Work out the finished part from the listing and answer in its coordinate system (mm). A direction names the side the tool comes from. Coordinates: 2 decimals unless noted, no trailing zeros. Order: outer loops, then holes, each group sorted by start corner. A loop starts at its lowest first (then second) coordinate and runs counter-clockwise, first axis right, second up. Notation, with made-up numbers: (5.5, -1) -> (11.5, -1) arc R13 cw to (11.5, 14) -> close; hole circle Ø4 at (58, 78.5). An arc over 180 degrees is marked (long way). Answer as CSV lines item,"result". Start each with the question number.
Item 1: For a pull along X with two mould halves and no side action, classify faces 3 (the face through (-46.315, 35, 3)), 4 (the face through (-43.315, 35, 4)), 5 (the face through (-42.315, 35, 4)), 6 (the face through (-43, 36, 6)) as pulls with the +X half, pulls with the -X half, needs draft (parallel to the pull), parting line crosses it, or undercut.
Item 2: Straight lines are drawn through the part: L1, parallel to X at y = 36, z = 5.55; L2, parallel to Z at x = -41.5, y = 36. For each, find the intervals that lie inside material, in ascending order.
Item 3: Section A-A (z = 5.5) is taken. Write down the section's boundary in (x, y), then the cut area to 3 significant figures.
Item 4: Which of the six approach directions +Z, -Z, +X, -X, +Y, -Y give full straight-line access (tool end or side, diameter ignored) to faces 1 (the face through (-35.815, 35, 4)), 2 (the face through (-32.815, 35, 3))?
Item 5: This flat-tipped pin is pushed along its axis until it touches: pin 1 Ø0.9 at (x, y) = (-41.5, 30) entering from +Z. Where does it stop, or does it pass through?
Item 6: Section B-B (y = 48.5) is taken. Write down the section's boundary in (x, z), then the cut area to 4 significant figures.
Item 7: Section C-C (x = -42) is taken. Write down the section's boundary in (y, z), then the cut area to 3 significant figures.
```python
from build123d import *

# Parameters (mm, degrees)
F0_W     = 100
F0_H     = 100
F1_DEPTH = 6
F2_W     = 2
F2_H     = 100
F2_W_2   = 1.75
F2_W_3   = 1.5
F2_W_4   = 1.25
F2_W_5   = 1
F3_DEPTH = 3.5
F4_W     = 86.5
F4_H     = 100
F5_DEPTH = 25
F6_W     = 13.5
F6_H     = 70
F7_DEPTH = 25


with BuildPart() as f1:
    # F0 (on Top) → F1 (new body)
    with BuildSketch(Plane.XY):
        with Locations((3.685346, 0.65935)):
            Rectangle(F0_W, F0_H)
    extrude(amount=F1_DEPTH)

    # F2 (on face) → F3 (cut)
    with BuildSketch(Plane.XY.offset(6)):
        with Locations((-44.314654, 0.65935)):
            Rectangle(F2_W, F2_H)
        with Locations((-41.439654, 0.65935)):
            Rectangle(F2_W_2, F2_H)
        with Locations((-38.814654, 0.65935)):
            Rectangle(F2_W_3, F2_H)
        with Locations((-36.439654, 0.65935)):
            Rectangle(F2_W_4, F2_H)
        with Locations((-34.314654, 0.65935)):
            Rectangle(F2_W_5, F2_H)
    extrude(amount=-F3_DEPTH, mode=Mode.SUBTRACT)

    # F4 (on face) → F5 (cut)
    with BuildSketch(Plane.XY.offset(6)):
        with Locations((10.435346, 0.65935)):
            Rectangle(F4_W, F4_H)
    extrude(amount=-F5_DEPTH, mode=Mode.SUBTRACT)

    # F6 (on face) → F7 (cut)
    with BuildSketch(Plane(origin=(0, 0, 0), x_dir=(1, 0, 0), z_dir=(0, 0, -1))):
        with Locations((-39.564654, 14.34065)):
            Rectangle(F6_W, F6_H)
    extrude(amount=-F7_DEPTH, mode=Mode.SUBTRACT)


solid = f1.part
```
Checked values:
1,face 3,"pulls with the -X half"
1,face 4,"undercut"
1,face 5,"undercut"
1,face 6,"needs draft"
2,L1,"x = -46.31 to -45.31, -43.31 to -42.31, -40.56 to -39.56, -38.06 to -37.06, -35.81 to -34.81, -33.81 to -32.81"
2,L2,"z = 0 to 2.5"
3,outline,"(-46.31, 20.66) -> (-45.31, 20.66) -> (-45.31, 50.66) -> (-46.31, 50.66) -> close; (-43.31, 20.66) -> (-42.31, 20.66) -> (-42.31, 50.66) -> (-43.31, 50.66) -> close; (-40.56, 20.66) -> (-39.56, 20.66) -> (-39.56, 50.66) -> (-40.56, 50.66) -> close; (-38.06, 20.66) -> (-37.06, 20.66) -> (-37.06, 50.66) -> (-38.06, 50.66) -> close; (-35.81, 20.66) -> (-34.81, 20.66) -> (-34.81, 50.66) -> (-35.81, 50.66) -> close; (-33.81, 20.66) -> (-32.81, 20.66) -> (-32.81, 50.66) -> (-33.81, 50.66) -> close"
3,area,"180 mm^2"
4,face 1,"+Z, +Y, -Y"
4,face 2,"+Z, -Z, +X, +Y, -Y"
5,pin 1,"stops at z = 2.5"
6,outline,"(-46.31, 0) -> (-32.81, 0) -> (-32.81, 6) -> (-33.81, 6) -> (-33.81, 2.5) -> (-34.81, 2.5) -> (-34.81, 6) -> (-35.81, 6) -> (-35.81, 2.5) -> (-37.06, 2.5) -> (-37.06, 6) -> (-38.06, 6) -> (-38.06, 2.5) -> (-39.56, 2.5) -> (-39.56, 6) -> (-40.56, 6) -> (-40.56, 2.5) -> (-42.31, 2.5) -> (-42.31, 6) -> (-43.31, 6) -> (-43.31, 2.5) -> (-45.31, 2.5) -> (-45.31, 6) -> (-46.31, 6) -> close"
6,area,"54.75 mm^2"
7,outline,"(20.66, 0) -> (50.66, 0) -> (50.66, 2.5) -> (20.66, 2.5) -> close"
7,area,"75.0 mm^2"
